Design review of the part built by this model. Coordinates are the model's own, in mm. A direction names the side the tool comes from. Give positions to 0.01 mm unless a question says otherwise; leave off trailing zeros. Loops run counter-clockwise (first coordinate to the right, second up) from the corner with the lowest first, then second, coordinate; pieces in that order, holes last.
Autodesk Inventor part; units mm, degrees
ref_plane "YZ Plane" through (0, 0, 0) normal (1, 0, 0) x (0, 1, 0)
ref_plane "XZ Plane" through (0, 0, 0) normal (0, 1, 0) x (-1, 0, 0)
ref_plane "XY Plane" through (0, 0, 0) normal (0, 0, 1) x (1, 0, 0)
sketch "Sketch1" plane through (0, 0, 0) normal (0, 1, 0) x (-1, 0, 0)
  line L0 (-21.4179, -39.4841) -> (-21.4179, -33.3379)
  line L1 (-21.4179, -33.3379) -> (-13.4169, -33.3379)
  line L2 (-13.4169, -33.3379) -> (-13.4169, -39.4841)
  line L3 (-13.4169, -39.4841) -> (-21.4179, -39.4841)
  line L4 (-21.4179, 41.7458) -> (-21.4179, 47.8919)
  line L5 (-21.4179, 47.8919) -> (-13.4169, 47.8919)
  line L6 (-13.4169, 47.8919) -> (-13.4169, 41.7458)
  line L7 (-13.4169, 41.7458) -> (-21.4179, 41.7458)
  circle A0 centre (-26.6249, -36.411) radius 3.175
  circle A1 centre (-26.6249, 44.8188) radius 3.175
  line L8 (-31.8319, 47.8919) -> (-31.8319, 41.7458)
  line L9 (-31.8319, 41.7458) -> (-39.8329, 41.7458)
  line L10 (-39.8329, 41.7458) -> (-39.8329, 47.8919)
  line L11 (-39.8329, 47.8919) -> (-31.8319, 47.8919)
  line L12 (-31.8319, -33.3379) -> (-31.8319, -39.4841)
  line L13 (-31.8319, -39.4841) -> (-39.8329, -39.4841)
  line L14 (-39.8329, -39.4841) -> (-39.8329, -33.3379)
  line L15 (-39.8329, -33.3379) -> (-31.8319, -33.3379)
  line L16 (-41.8649, 3.1879) -> (-27.6409, 3.1879)
  line L17 (-27.6409, 3.1879) -> (-27.6409, -6.9721)
  line L18 (-27.6409, -6.9721) -> (-41.8649, -6.9721)
  line L19 (-41.8649, -6.9721) -> (-41.8649, -9.0041)
  line L20 (-41.8649, -9.0041) -> (-27.6409, -9.0041)
  line L21 (-27.6409, -9.0041) -> (-27.6409, -19.1641)
  line L22 (-27.6409, -19.1641) -> (-41.8649, -19.1641)
  line L23 (-41.8649, -19.1641) -> (-41.8649, -21.1961)
  line L24 (-41.8649, -21.1961) -> (-27.6409, -21.1961)
  line L25 (-27.6409, -21.1961) -> (-27.6409, -31.3561)
  line L26 (-27.6409, -31.3561) -> (-41.8649, -31.3561)
  line L27 (-41.8649, -31.3561) -> (-41.8649, -41.5161)
  line L28 (-41.8649, -41.5161) -> (-11.3849, -41.5161)
  line L29 (-11.3849, -41.5161) -> (-11.3849, -31.3561)
  line L30 (-11.3849, -31.3561) -> (-25.6089, -31.3561)
  line L31 (-25.6089, -31.3561) -> (-25.6089, -21.1961)
  line L32 (-25.6089, -21.1961) -> (-11.3849, -21.1961)
  line L33 (-11.3849, -21.1961) -> (-11.3849, -19.1641)
  line L34 (-11.3849, -19.1641) -> (-25.6089, -19.1641)
  line L35 (-25.6089, -19.1641) -> (-25.6089, -9.0041)
  line L36 (-25.6089, -9.0041) -> (-11.3849, -9.0041)
  line L37 (-11.3849, -9.0041) -> (-11.3849, -6.9721)
  line L38 (-11.3849, -6.9721) -> (-25.6089, -6.9721)
  line L39 (-25.6089, -6.9721) -> (-25.6089, 3.1879)
  line L40 (-25.6089, 3.1879) -> (-11.3849, 3.1879)
  line L41 (-11.3849, 3.1879) -> (-11.3849, 5.2199)
  line L42 (-11.3849, 5.2199) -> (-25.6089, 5.2199)
  line L43 (-25.6089, 5.2199) -> (-25.6089, 15.3799)
  line L44 (-25.6089, 15.3799) -> (-11.3849, 15.3799)
  line L45 (-11.3849, 15.3799) -> (-11.3849, 17.4119)
  line L46 (-11.3849, 17.4119) -> (-25.6089, 17.4119)
  line L47 (-25.6089, 17.4119) -> (-25.6089, 27.5719)
  line L48 (-25.6089, 27.5719) -> (-11.3849, 27.5719)
  line L49 (-11.3849, 27.5719) -> (-11.3849, 29.6039)
  line L50 (-11.3849, 29.6039) -> (-25.6089, 29.6039)
  line L51 (-25.6089, 29.6039) -> (-25.6089, 39.7639)
  line L52 (-25.6089, 39.7639) -> (-11.3849, 39.7639)
  line L53 (-11.3849, 39.7639) -> (-11.3849, 49.9239)
  line L54 (-11.3849, 49.9239) -> (-41.8649, 49.9239)
  line L55 (-41.8649, 49.9239) -> (-41.8649, 39.7639)
  line L56 (-41.8649, 39.7639) -> (-27.6409, 39.7639)
  line L57 (-27.6409, 39.7639) -> (-27.6409, 29.6039)
  line L58 (-27.6409, 29.6039) -> (-41.8649, 29.6039)
  line L59 (-41.8649, 29.6039) -> (-41.8649, 27.5719)
  line L60 (-41.8649, 27.5719) -> (-27.6409, 27.5719)
  line L61 (-27.6409, 27.5719) -> (-27.6409, 17.4119)
  line L62 (-27.6409, 17.4119) -> (-41.8649, 17.4119)
  line L63 (-41.8649, 17.4119) -> (-41.8649, 15.3799)
  line L64 (-41.8649, 15.3799) -> (-27.6409, 15.3799)
  line L65 (-27.6409, 15.3799) -> (-27.6409, 5.2199)
  line L66 (-27.6409, 5.2199) -> (-41.8649, 5.2199)
  line L67 (-41.8649, 5.2199) -> (-41.8649, 3.1879)
  line L68 (-11.3849, -31.3561) -> (-11.3849, 39.7639)
  line L69 (-41.8649, 39.7639) -> (-41.8649, -31.3561)
  point P0 (0, 0)
extrude "Extrusion1" add sketch "Sketch1" along normal blind 2.54 contours L0 L1 L2 L3 | L4 L5 L6 L7 | L8 L9 L10 L11 | L12 L13 L14 L15 | L67 L66 L65 L64 L63 L62 L61 L60 L59 L58 L57 L56 L55 L54 L53 L52 L51 L50 L49 L48 L47 L46 L45 L44 L43 L42 L41 L40 L39 L38 L37 L36 L35 L34 L33 L32 L31 L30 L29 L28 L27 L26 L25 L24 L23 L22 L21 L20 L19 L18 L17 L16 | L16 L17 L18 L69 | L69 L64 L65 L66 | L20 L21 L22 L69 | L69 L60 L61 L62 | L24 L25 L26 L69 | L69 L56 L57 L58 | L30 L31 L32 L68 | L68 L50 L51 L52 | L34 L35 L36 L68 | L68 L46 L47 L48 | L38 L39 L40 L68 | L68 L42 L43 L44
chamfer "Chamfer1" distance 2.54 angle 45 4 edges at (26.6249, 2.54, 49.9239) (41.8649, 2.54, -20.1801) (11.3849, 2.54, -36.4361) (26.6249, 2.54, -41.5161)
sketch "Sketch2" plane through (0, 0, 0) normal (0, -1, 0) x (1, 0, 0)
  circle A0 centre (26.6249, 44.8188) radius 3.175
  circle A1 centre (26.6249, 44.8188) radius 3.175
  circle A2 centre (26.6249, -36.411) radius 3.175
  circle A3 centre (26.6249, -36.411) radius 3.175
  point P0 (0, 0)
extrude "Extrusion2" add sketch "Sketch2" along normal blind 2.54
sketch "Sketch3" plane through (26.6249, 0, 44.8188) normal (0, 1, 0) x (1, 0, 0)
  circle A0 centre (0, 81.2298) radius 3.175
  circle A1 centre (0, 0) radius 3.175
  point P0 (-26.6249, 44.8188)
extrude "Extrusion3" add sketch "Sketch3" along normal blind 2.54
sketch "Sketch4" plane through (11.3849, 0, 49.9239) normal (0, 0.7071068, 0.7071068) x (1, 0, 0)
  line L0 (10.0398, 1.9622) -> (22.6044, 1.9622)
  line L1 (22.6044, 1.9622) -> (22.6044, 6.858)
  line L2 (22.6044, 6.858) -> (10.0398, 6.858)
  line L3 (10.0398, 6.858) -> (10.0398, 1.9622)
  point P0 (-11.3849, 35.3015)
extrude "Extrusion4" cut sketch "Sketch4" along normal blind 2.54
sketch "Sketch5" plane through (41.8649, 0, -41.5161) normal (0, 0.7071068, -0.7071068) x (-1, 0, 0)
  line L0 (9.9656, 2.1621) -> (20.0479, 2.1621)
  line L1 (20.0479, 2.1621) -> (20.0479, 4.6266)
  line L2 (20.0479, 4.6266) -> (9.9656, 4.6266)
  line L3 (9.9656, 4.6266) -> (9.9656, 2.1621)
  point P0 (41.8649, 29.3563)
extrude "Extrusion5" cut sketch "Sketch5" along normal blind 2.54
properties part number "TerminalBlockLid"
Q1. Take a section at C-C (y = -1.35). Give the boundary of the cut face in (x, z) (3 decimals).
Results:
outline: circle Ø6.35 at (26.625, -36.411); circle Ø6.35 at (26.625, 44.819)
Q2. Take a section at B-B (z = -13). Give the boundary of the cut face in (x, y), plus the area to 3 significant figures.
Results:
outline: (11.38, 0) - (41.86, 0) - (39.32, 2.54) - (13.92, 2.54) - close
area: 71.0 mm2
Q3. Tool access review of faces 1 (the face through (25.94, -1.25, -33.31)), 2 (the face through (27, 2.54, 5)): name each direction out of +Z, -Z, +X, -X, +Y, -Y from which nothing blocks a thin tool from reaching the whole face with its end or side.
Results:
face 1: -Y
face 2: +Z, -Z, +X, -X, +Y
Q4. Wall thickness on line 1 (Y direction, x = 36, z = -2); line 2 (X direction, y = 1, z = 9); line 3 (X direction, y = 0.7, z = 40): over which ranges is each line inside the solid? List them lowest first.
Results:
line 1: y = 0 to 2.54
line 2: x = 12.38 to 40.86
line 3: x = 12.08 to 41.16
Q5. Take a section at D-D (x = 38). Give the boundary of the cut face in (y, z).
Results:
outline: (0, -41.52) - (2.54, -38.98) - (2.54, 47.38) - (0, 49.92) - close
Q6. Insertion check: pin 1 (0.8 mm diameter, centred on y = 2, z = -39.5, fed in from -X); pin 2 (0.9 mm diameter, centred on y = 2, z = 48, fed in from -X); pin 3 (1.3 mm diameter, centred on y = 2, z = 48, fed in from +X). Each pin has a flat end and moves straight along its axis. Give the tip position at first contact, or say it passes through.
Results:
pin 1: stops at x = 12.98
pin 2: stops at x = 12.93
pin 3: stops at x = 40.51
